The listing builds one solid part. Answer for the finished solid, in the listing's coordinates (mm). Face numbers are marked on the shaded views. A direction names the side the tool comes from. Round coordinates to 2 decimals unless told otherwise and drop trailing zeros. Order: outer loops, then holes, each group sorted by start corner. A loop starts at its lowest first (then second) coordinate and runs counter-clockwise, first axis right, second up. Notation, with made-up numbers: (82, 5.25) - (124, 5.25) arc R18 cw to (124, 31.25) - close; hole circle Ø9 at (49.5, 85.5). An arc over 180 degrees is marked (long way). One line per item, written item: value. Start each with the question number.
1. Section A-A, the plane z = 13.5 is taken. Give the vertices of the cut face in (x, y).
2. A tool of negligible diameter and unlimited length cuts with its end or side. For the marked faces 1, 2 and 3, from which of +Z, -Z, +X, -X, +Y, -Y can it reach the whole face along a straight path? Write none if from no direction.
3. Flat-ended cylindrical pins translate along their axes: P1, Ø3, axis at x = 92.5, z = 10, coming from the -Y side; P2, Ø4.5, axis at x = 7, y = 0, coming from the -Z side; P3, Ø2, axis at x = 45.5, y = 1, coming from the -Z side; P4, Ø1, axis at x = 59.5, z = 16, coming from the +Y side. Find the tip coordinate at first contact, or state that the pin passes through.
4. Straight lines are drawn through the part: line 1 (X direction, y = 0, z = 1.6); line 2 (Y direction, x = 12.5, z = 16.5); line 3 (Y direction, x = 0, z = 2.65). For each, find the intervals that lie inside material, in ascending order.
5. Section B-B, the plane x = 57 is taken. Give the vertices of the cut face in (y, z), then the cut area to 3 significant figures.
from build123d import *

# Parameters (mm, degrees)
SKETCH1_R               = 13
ELBOW_BOSS_DEPTH        = 19
BAR_DEPTH               = 19
CUT_EXTRUDE1_DEPTH      = 133.022725317
CUT_EXTRUDE1_DEPTH_BACK = 4
SKETCH3_R               = 10.1
SKETCH4_R               = 4.25
CUT_EXTRUDE2_DEPTH      = 2.6
SKETCH5_R               = 2
CUT_EXTRUDE3_DEPTH      = 10
SKETCH6_R               = 2
CUT_EXTRUDE4_DEPTH      = 13
SKETCH7_R               = 1.1
CUT_EXTRUDE5_DEPTH      = 132.506653824
CIRPATTERN1_COUNT       = 4


with BuildPart() as part:
    # Sketch1 → Elbow Boss (new body)
    with BuildSketch(Plane.XY):
        Circle(SKETCH1_R)
    extrude(amount=ELBOW_BOSS_DEPTH)

    # Sketch2 → Bar (add)
    with BuildSketch(Plane.XY):
        with BuildLine():
            Line((0, 10), (120, 10))
            ThreePointArc((120, 10), (130, 0), (120, -10))
            Line((120, -10), (0, -10))
            ThreePointArc((0, -10), (-10, 0), (0, 10))
        make_face()
    extrude(amount=BAR_DEPTH)

    # Sketch3 → Cut-Extrude1 (cut, two sides: drawn at the far end of the back side and taken through both)
    with BuildSketch(Plane(origin=(0, 0, 0), x_dir=(-1, 0, 0), z_dir=(0, 0, -1)).offset(-CUT_EXTRUDE1_DEPTH_BACK)):
        Circle(SKETCH3_R)
    extrude(amount=CUT_EXTRUDE1_DEPTH + CUT_EXTRUDE1_DEPTH_BACK, mode=Mode.SUBTRACT)

    # Sketch4 → Cut-Extrude2 (cut)
    with BuildSketch(Plane(origin=(0, 0, 4), x_dir=(-1, 0, 0), z_dir=(0, 0, -1))):
        Circle(SKETCH4_R)
    extrude(amount=-CUT_EXTRUDE2_DEPTH, mode=Mode.SUBTRACT)

    # Sketch5 → Cut-Extrude3 (cut)
    with BuildSketch(Plane.XY.offset(19)):
        Circle(SKETCH5_R)
    extrude(amount=-CUT_EXTRUDE3_DEPTH, mode=Mode.SUBTRACT)

    # Sketch6 → Cut-Extrude4 (cut)
    with BuildSketch(Plane.XY.offset(19)):
        with Locations((7, 0)):
            Circle(SKETCH6_R)
    cut_extrude4 = extrude(amount=-CUT_EXTRUDE4_DEPTH, mode=Mode.SUBTRACT)

    # Sketch7 → Cut-Extrude5 (cut, through all)
    with BuildSketch(Plane(origin=(0, 0, 4), x_dir=(-1, 0, 0), z_dir=(0, 0, -1))):
        with Locations((-7, 0)):
            Circle(SKETCH7_R)
    cut_extrude5 = extrude(amount=-CUT_EXTRUDE5_DEPTH, mode=Mode.SUBTRACT)

    # CirPattern1: Cut-Extrude4, Cut-Extrude5 ×4 about axis
    cirpattern1_axis = Axis((0, 0, 0), (0, 0, 1))
    add([cut_extrude4.rotate(cirpattern1_axis, i * 360 / CIRPATTERN1_COUNT) for i in range(1, CIRPATTERN1_COUNT)], mode=Mode.SUBTRACT)
    add([cut_extrude5.rotate(cirpattern1_axis, i * 360 / CIRPATTERN1_COUNT) for i in range(1, CIRPATTERN1_COUNT)], mode=Mode.SUBTRACT)


solid = part.part
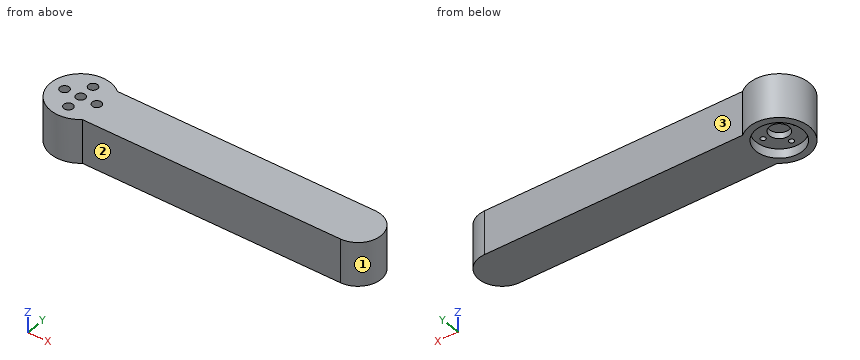
Answer list:
1. outline: (8.31, -10) - (120, -10) arc R10 ccw to (120, 10) - (8.31, 10) arc R13 ccw (long way) to start; hole circle Ø4 at (-7, 0); hole circle Ø4 at (0, -7); hole circle Ø4 at (0, 0); hole circle Ø4 at (0, 7); hole circle Ø4 at (7, 0)
2. face 1: +Z, -Z, +X
2. face 2: +Z, -Z, +X, -Y
2. face 3: +Z, -Z, +X, +Y
3. P1: stops at y = -10
3. P2: stops at z = 4
3. P3: stops at z = 0
3. P4: stops at y = 10
4. line 1: x = -13 to -10.1, 10.1 to 130
4. line 2: y = -10 to 10
4. line 3: y = -13 to -10.1, 10.1 to 13
5. outline: (-10, 0) - (10, 0) - (10, 19) - (-10, 19) - close
5. area: 380 mm²
